Source: CAD feature listing. Evaluate the final solid. Frame: model axes, mm. A direction names the side the tool comes from. Give positions to 0.01 mm unless a question says otherwise; leave off trailing zeros. Loops run counter-clockwise (first coordinate to the right, second up) from the corner with the lowest first, then second, coordinate; pieces in that order, holes last. Notation, with made-up numbers: M 7,-9.75 L 57,-9.75 A32 cw 57,25.25 Z; hole C -19,42.25 d5. An arc over 180 degrees is marked long. Write item = value, one per line.
from build123d import *

# Parameters (mm, degrees)
F0_R     = 2.54
F1_DEPTH = 23.4442
F3_D     = 18.288
F3_DEPTH = 16.51
F3_TIP   = 5.4942695004
F5_DEPTH = 101.6
F7_D     = 17.78
F7_DEPTH = 114.3
F7_TIP   = 5.3416509032
F8_R     = 5.08


with BuildPart() as f1:
    # F0 (on Front) → F1 (new body)
    with BuildSketch(Plane.XZ):
        Polygon((14.5139638376, 46.979337565), (6.0992269906, 54.9012346102), (-6.9395108012, 52.6397765944), (-19.2585108012, 31.302642696), (-19.2585108012, 20.126642696), (0.6639761268, 20.126642696), (12.2374891988, 20.126642696), (12.2374891988, 39.176642696), align=None)
        with Locations((-13.805717687, 25.5267831615)):
            Circle(F0_R, mode=Mode.SUBTRACT)
        with Locations((3.3416109761, 50.2072100538)):
            Circle(F0_R, mode=Mode.SUBTRACT)
    extrude(amount=F1_DEPTH)

    # F3
    with Locations(Plane.XZ.offset(23.4442)):
        with Locations((-0.7346722452, 36.7999244481)):
            Hole(F3_D / 2, depth=F3_DEPTH)
            with Locations((0, 0, -(F3_DEPTH + F3_TIP / 2))):  # 118° drill point
                Cone(0, F3_D / 2, F3_TIP, mode=Mode.SUBTRACT)

    # F4 (on face) → F5 (join)
    with BuildSketch(Plane(origin=(0, 0, 20.126642696), x_dir=(1, 0, 0), z_dir=(0, 0, -1))):
        with BuildLine():
            ThreePointArc((-2.5011187059, 0), (3.9646657012, 2.6782155928), (6.6428812941, 9.144))
            ThreePointArc((6.6428812941, 9.144), (-8.9669031131, 15.6097844072), (-2.5011187059, 0))
        make_face()
    extrude(amount=F5_DEPTH)

    # F7
    with Locations(Plane(origin=(0, 0, -81.473357304), x_dir=(1, 0, 0), z_dir=(0, 0, -1))):
        with Locations((-2.5011187059, 9.144)):
            Hole(F7_D / 2, depth=F7_DEPTH)
            with Locations((0, 0, -(F7_DEPTH + F7_TIP / 2))):  # 118° drill point
                Cone(0, F7_D / 2, F7_TIP, mode=Mode.SUBTRACT)

    # F8
    f8_edges = [f1.edges().sort_by_distance(p)[0] for p in [
        (6.099227, -11.7221, 54.901235),
        (14.513964, -11.7221, 46.979338),
        (12.237489, -11.7221, 20.126643),
        (-19.258511, -11.7221, 20.126643),
        (-6.939511, -11.7221, 52.639777),
        (-19.258511, -11.7221, 31.302643),
    ]]
    fillet(f8_edges, radius=F8_R)


solid = f1.part
1. Cut plane B-B, the plane z = -60. Return the cut outline in (x, y), then the cut area to 3 significant figures.
Derived:
outline = C -2.5,-9.14 d18.29; hole C -2.5,-9.14 d17.78
area = 14.4 mm²
2. Cut plane C-C, the plane x = 10.5. Return the cut outline in (y, z), then the cut area to 3 significant figures.
Derived:
outline = M -23.44,21.38 L 0,21.38 L 0,50.76 L -23.44,50.76 Z
area = 689 mm²
3. First-contact query: pin 1 Ø1 at (x, y) = (1.5, -6) entering from +Z; pin 2 Ø12 at (y, z) = (-8.5, -7) entering from -X; pin 3 Ø12 at (x, z) = (-15, -54) entering from -Y. Flat tips, straight axial feed; report the tip coordinate or a pass-through.
Derived:
pin_1 = 54.19
pin_2 = -11.65
pin_3 = -15.58
4. Material intervals for probe 1 along X at (y, z) = (-9.25, -12); probe 2 along Z at (x, y) = (7.5, -9.75); probe 3 along Y at (x, z) = (-9, -40), sorted ascending. Write a range as from..to.
Derived:
probe_1 = -11.64..-11.39, 6.39..6.64
probe_2 = 20.14..32.82, 40.78..53.54
probe_3 = -15.58..-15.21, -3.08..-2.71
5. Pull-direction query (X, two-part tool) for faces 1 (the flat face through (-10, -23.444, 34)), 2 (the conical face through (-5.627, -4.376, 34.743)), 3 (the flat face through (-13.28, -11.56, 41.66)); classes: +X half, -X half, draft (parallel to the pull), parting line (faces both ways), or undercut.
Derived:
face_1 = draft
face_2 = undercut
face_3 = -X half
6. Cut plane A-A, the plane y = -16.5. Return the cut outline in (x, z).
Derived:
outline = M -19.26,25.21 A5.08 ccw -14.18,20.13 L -7.93,20.13 L -7.93,-81.47 L -7.49,-81.47 L -7.49,30.64 A9.14 cw long 2.49,28.24 L 2.49,-81.47 L 2.93,-81.47 L 2.93,20.13 L 7.16,20.13 A5.08 ccw 12.24,25.21 L 12.24,39.18 L 13.64,43.99 A5.08 ccw 12.25,49.11 L 7.95,53.16 A5.08 ccw 3.6,54.47 L -4.6,53.05 A5.08 ccw -8.13,50.58 L -18.58,32.48 A5.08 ccw -19.26,29.94 Z; hole C -13.81,25.53 d5.08; hole C 3.34,50.21 d5.08
7. Reachability of faces 4 (the flat face through (12.237, -12, 32)), 5 (the flat face through (-8, -17, 20.127)), 6 (the cylindrical face through (0.456, -15.074, 45.866)) from +Z, -Z, +X, -X, +Y, -Y: full face, straight path, thin tool, end or side. Return the list, or none.
Derived:
face_4 = -Z, +X, +Y, -Y
face_5 = -Z
face_6 = -Y
